```python
from build123d import *

# Parameters (mm, degrees)
PAD_DEPTH       = 38.6
POCKET_DEPTH    = 16
POCKET001_DEPTH = 23
POCKET002_DEPTH = 14


with BuildPart() as part:
    # Sketch → Pad (new body)
    with BuildSketch(Plane.YZ):
        with BuildLine():
            Line((0, 0), (34.2, 0))
            Line((34.2, 0), (34.2, 32.8))
            ThreePointArc((34.2, 32.8), (33.32132, 34.92132), (31.2, 35.8))
            Line((31.2, 35.8), (3, 35.8))
            ThreePointArc((3, 35.8), (0.87868, 34.92132), (0, 32.8))
            Line((0, 32.8), (0, 0))
        make_face()
    extrude(amount=PAD_DEPTH)

    # Sketch001 (on Face7 of Pad) → Pocket (cut)
    with BuildSketch(Plane(origin=(0, 0, 0), x_dir=(0, 1, 0), z_dir=(-1, 0, 0))):
        Polygon((4, -3), (4, -1), (29, -1), (29, -3), (32.2, -3), (32.2, -5.5), (29, -5.5), (29, -7.5), (4, -7.5), (4, -5.5), (1, -5.5), (1, -3), align=None)
    extrude(amount=-POCKET_DEPTH, mode=Mode.SUBTRACT)

    # Sketch002 (on Face5 of Pocket) → Pocket001 (cut)
    with BuildSketch(Plane.YZ.offset(38.6)):
        with BuildLine():
            Line((1, 1), (33.2, 1))
            Line((33.2, 1), (33.2, 31.8))
            ThreePointArc((33.2, 31.8), (32.32132, 33.92132), (30.2, 34.8))
            Line((30.2, 34.8), (4, 34.8))
            ThreePointArc((4, 34.8), (1.87868, 33.92132), (1, 31.8))
            Line((1, 31.8), (1, 1))
        make_face()
    extrude(amount=-POCKET001_DEPTH, mode=Mode.SUBTRACT)

    # Sketch003 (on Face29 of Pocket001) → Pocket002 (cut)
    with BuildSketch(Plane.YZ.offset(15.6)):
        with BuildLine():
            Line((1, 7.5), (33.273769, 7.5))
            Line((33.273769, 7.5), (33.273769, 31.8))
            ThreePointArc((33.273769, 31.8), (32.395089, 33.92132), (30.273769, 34.8))
            Line((30.273769, 34.8), (4, 34.8))
            ThreePointArc((4, 34.8), (1.87868, 33.92132), (1, 31.8))
            Line((1, 31.8), (1, 7.5))
        make_face()
    extrude(amount=-POCKET002_DEPTH, mode=Mode.SUBTRACT)


solid = part.part
```
Here's how the part is built. I have some questions about the finished solid (model axes, mm). A direction names the side the tool comes from. Round coordinates to 2 decimals unless told otherwise and drop trailing zeros. Loops run counter-clockwise (first coordinate to the right, second up) from the corner with the lowest first, then second, coordinate; pieces in that order, holes last.
1. Suppose I cut it at B-B, the plane x = 10.5. Please give me the cut outline in (y, z), and give its area (3 significant figures).
Answers:
outline: (0, 0) - (34.2, 0) - (34.2, 32.8) arc R3 ccw to (31.2, 35.8) - (3, 35.8) arc R3 ccw to (0, 32.8) - close; hole (1, 3) - (4, 3) - (4, 1) - (29, 1) - (29, 3) - (32.2, 3) - (32.2, 5.5) - (29, 5.5) - (29, 7.5) - (33.27, 7.5) - (33.27, 31.8) arc R3 ccw to (30.27, 34.8) - (4, 34.8) arc R3 ccw to (1, 31.8) - (1, 7.5) - (4, 7.5) - (4, 5.5) - (1, 5.5) - close
area: 165 mm2
2. Will these pins go through, and if not, where does the flat tip stop? pin 1 (2 mm diameter, centred on y = 3, z = 7, fed in from +X); pin 2 (13.5 mm diameter, centred on y = 21.5, z = 27, fed in from +X).
Answers:
pin 1: stops at x = 15.6
pin 2: stops at x = 1.6
3. If I drill on probe 1 along Z at (x, y) = (27, 12.5); probe 2 along Y at (x, z) = (26, 24.5); probe 3 along Z at (x, y) = (4.5, 2.5), over which ranges is the centre line in solid material (lowest first)?
Answers:
probe 1: z = 0 to 1, 34.8 to 35.8
probe 2: y = 0 to 1, 33.2 to 34.2
probe 3: z = 0 to 3, 5.5 to 7.5, 34.4 to 35.76
4. Thinking about a two-plate mould opening in Y: for faces 6 (the face through (38.6, 0.6, 18)), 7 (the face through (8, 31, 5.5)), 8 (the face through (19.03, 0.9, 34.94)), 9 (the face through (19, 34.2, 16)), which applies, released by +Y, released by -Y, zero draft, split by the parting line, or undercut?
Answers:
face 6: zero draft
face 7: undercut
face 8: released by -Y
face 9: released by +Y
5. Suppose I cut it at D-D, the plane z = 28.5. Please give me the cut outline in (x, y).
Answers:
outline: (0, 0) - (38.6, 0) - (38.6, 1) - (1.6, 1) - (1.6, 33.27) - (15.6, 33.27) - (15.6, 33.2) - (38.6, 33.2) - (38.6, 34.2) - (0, 34.2) - close
6. Suppose I cut it at A-A, the plane z = 4. Please give me the cut outline in (x, y).
Answers:
outline: (0, 0) - (38.6, 0) - (38.6, 1) - (0, 1) - close; (0, 32.2) - (15.6, 32.2) - (15.6, 33.2) - (38.6, 33.2) - (38.6, 34.2) - (0, 34.2) - close
7. Suppose I cut it at C-C, the plane y = 23. Please give me the cut outline in (x, z).
Answers:
outline: (0, 0) - (38.6, 0) - (38.6, 1) - (0, 1) - close; (0, 7.5) - (1.6, 7.5) - (1.6, 34.8) - (38.6, 34.8) - (38.6, 35.8) - (0, 35.8) - close
8. For faces 1 (the face through (20.36, 1.9, 33.94)), 2 (the face through (8, 29, 6)), 3 (the face through (9, 33.274, 19)), 4 (the face through (19, 0, 17)), 5 (the face through (19, 17, 0)), which set-ups out of +Z, -Z, +X, -X, +Y, -Y let a thin tool reach every point of the face, with its end or its side?
Answers:
face 1: +X
face 2: +X, -X
face 3: none
face 4: +Z, -Z, +X, -X, -Y
face 5: -Z, +X, -X, +Y, -Y
